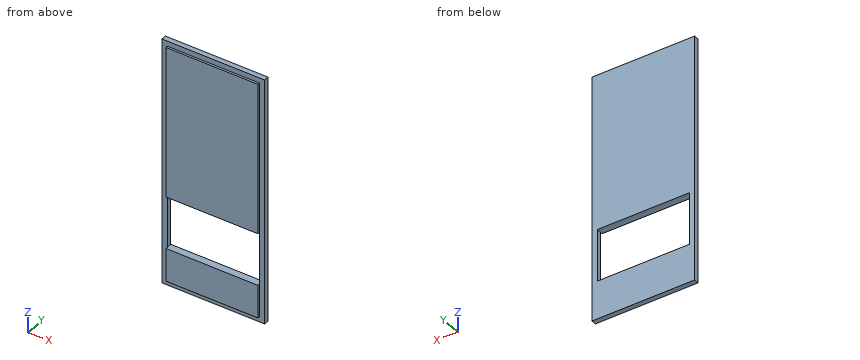
```python
from build123d import *

# Parameters (mm, degrees)
SKETCH1_W           = 26
SKETCH1_H           = 68
BOSS_EXTRUDE1_DEPTH = 0.6
SKETCH2_W           = 29
SKETCH2_H           = 71
BOSS_EXTRUDE2_DEPTH = 1.4
SKETCH3_W           = 26
SKETCH3_H           = 15
CUT_EXTRUDE1_DEPTH  = 15.4


with BuildPart() as part:
    # Sketch1 → Boss-Extrude1 (new body)
    with BuildSketch(Plane(origin=(0, 11.5, 0), x_dir=(1, 0, 0), z_dir=(0, 1, 0))):
        with Locations((14.5, 35.5)):
            Rectangle(SKETCH1_W, SKETCH1_H)
    extrude(amount=-BOSS_EXTRUDE1_DEPTH)

    # Sketch2 → Boss-Extrude2 (add)
    with BuildSketch(Plane(origin=(0, 11.5, 0), x_dir=(1, 0, 0), z_dir=(0, 1, 0))):
        with Locations((14.5, 35.5)):
            Rectangle(SKETCH2_W, SKETCH2_H)
    extrude(amount=BOSS_EXTRUDE2_DEPTH)

    # Sketch3 → Cut-Extrude1 (cut)
    with BuildSketch(Plane.XZ.offset(-10.9)):
        with Locations((14.5, -52.5)):
            Rectangle(SKETCH3_W, SKETCH3_H)
    extrude(amount=-CUT_EXTRUDE1_DEPTH, mode=Mode.SUBTRACT)


solid = part.part
```
The listing builds one solid part. Answer for the finished solid, in the listing's coordinates (mm). Give positions to 0.01 mm unless a question says otherwise; leave off trailing zeros. Order: outer loops, then holes, each group sorted by start corner. A loop starts at its lowest first (then second) coordinate and runs counter-clockwise, first axis right, second up. Notation, with made-up numbers: (71, 43.25) -> (93, 43.25) arc R13 cw to (93, 49.25) -> close; hole circle Ø4 at (-1.75, 36). An arc over 180 degrees is marked (long way). Answer as CSV lines item,"result". Start each with the question number.
Q1. A cutting plane is placed at C-C (z = -26). Determine the outline of the cut face in (x, y), then the cut area to 3 significant figures.
Q2. A cutting plane is placed at A-A (y = 12.1). Determine the outline of the cut face in (x, z).
Q3. Given pin 1 (0.7 mm diameter, centred on x = 10.5, y = 11, fed in from +Z); pin 2 (0.7 mm diameter, centred on y = 11, z = -65, fed in from -X); pin 3 (8.5 mm diameter, centred on x = 13, z = -52.5, fed in from -Y), each flat-ended and moving along its own axis, determine where each tip first touches the part or whether it passes through.
Q4. Find the intervals of material crossed by L1, parallel to Z at x = 7.25, y = 11.9; L2, parallel to Z at x = 3.25, y = 11.45; L3, parallel to X at y = 12.05, z = -49, in increasing order.
Q5. A cutting plane is placed at B-B (x = 8). Determine the outline of the cut face in (y, z), then the cut area to 3 significant figures.
Results found:
1,outline,"(0, 11.5) -> (1.5, 11.5) -> (1.5, 10.9) -> (27.5, 10.9) -> (27.5, 11.5) -> (29, 11.5) -> (29, 12.9) -> (0, 12.9) -> close"
1,area,"56.2 mm2"
2,outline,"(0, -71) -> (29, -71) -> (29, 0) -> (0, 0) -> close; hole (1.5, -60) -> (27.5, -60) -> (27.5, -45) -> (1.5, -45) -> close"
3,pin 1,"z = -1.5"
3,pin 2,"x = 1.5"
3,pin 3,"through"
4,L1,"-71 to -60, -45 to 0"
4,L2,"-69.5 to -60, -45 to -1.5"
4,L3,"0 to 1.5, 27.5 to 29"
5,outline,"(10.9, -69.5) -> (11.5, -69.5) -> (11.5, -71) -> (12.9, -71) -> (12.9, -60) -> (10.9, -60) -> close; (10.9, -45) -> (12.9, -45) -> (12.9, 0) -> (11.5, 0) -> (11.5, -1.5) -> (10.9, -1.5) -> close"
5,area,"110 mm2"
